Answer from the drawing. Dimensions are ordinates in mm from the lowest x, y and z of the part. Give positions to 0.01 mm unless a question says otherwise; leave off trailing zeros. Write each loop counter-clockwise with the first axis right and the second up, starting at its lowest first coordinate (ties: lowest second). Pieces come first, ordered by that corner, then holes. Notation, with made-up numbers: M -39.75,16.25 L -26.75,16.25 A10 ccw -26.75,32.25 Z; hole C 1,39.25 d6. An arc over 180 degrees is marked long. Answer as a JSON object with one key per item and string values.
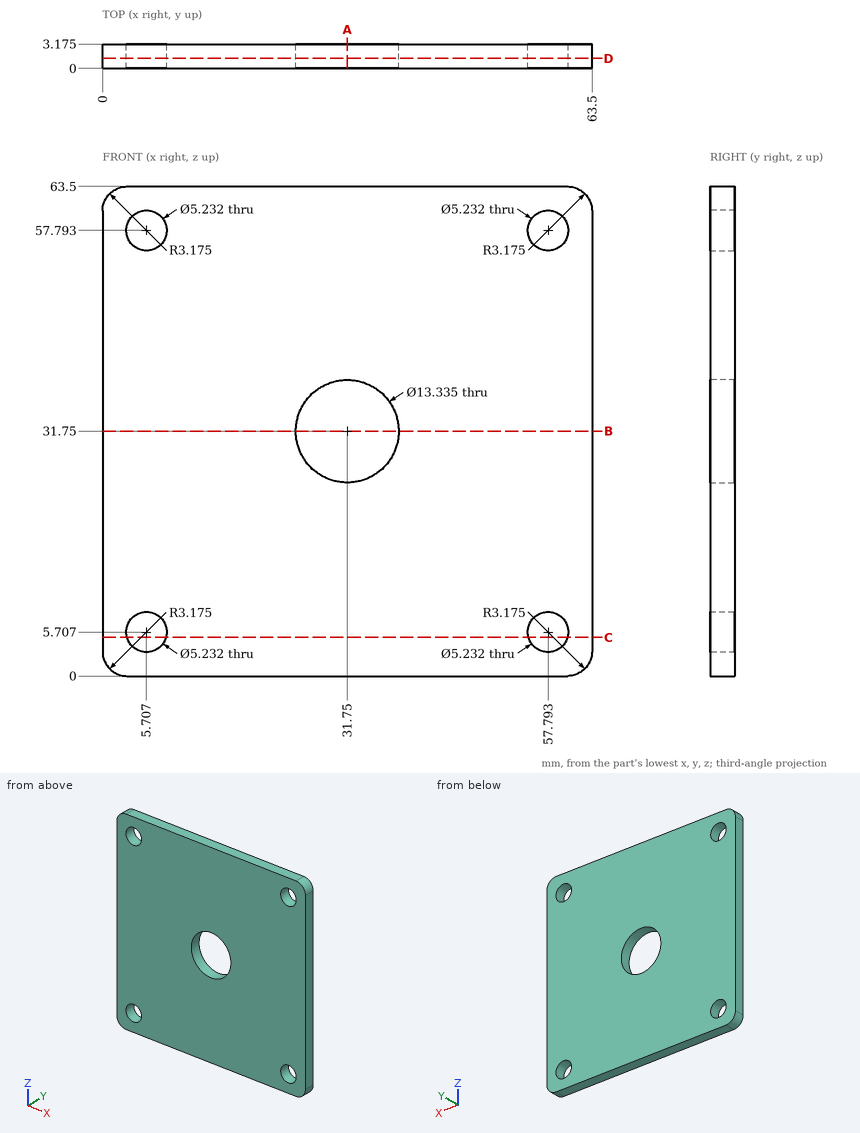
1. A cutting plane is placed at C-C, the plane z = 5. Give the vertices of the cut face in (x, y) (1 decimal).
Verdict:
{"outline": "M 0,0 L 3.2,0 L 3.2,3.2 L 0,3.2 Z; M 8.2,0 L 55.3,0 L 55.3,3.2 L 8.2,3.2 Z; M 60.3,0 L 63.5,0 L 63.5,3.2 L 60.3,3.2 Z"}
2. Consider line 1 along X through (y, z) = (0.2, 31.5); line 2 along Z through (x, y) = (7.5, 0.15) (1 decimal); line 3 along X through (y, z) = (1.1, 7). Determine where each line is inside the solid, lowest interval first.
Verdict:
{"line 1": "x = 0 to 25.09, 38.41 to 63.5", "line 2": "z = 0 to 3.8, 7.6 to 55.9, 59.7 to 63.5", "line 3": "x = 0 to 3.43, 7.98 to 55.52, 60.07 to 63.5"}
3. A cutting plane is placed at D-D, the plane y = 1.3. Count the separate pieces of the cut face and the enclosed holes in it, plus the area to 3 significant figures.
Verdict:
{"separate pieces": "1", "enclosed holes": "5", "area": "3,800 mm2"}
4. A flat-ended cylindrical pin translates along its axis: pin 1 (4 mm diameter, centred on x = 57.79, z = 5.71, fed in from -Y). Find the tip coordinate at first contact, or state that the pin passes through.
Verdict:
{"pin 1": "passes through"}
5. A cutting plane is placed at A-A, the plane x = 31.75. Give the vertices of the cut face in (y, z) (1 decimal), plus the area to 3 significant figures.
Verdict:
{"outline": "M 0,0 L 3.2,0 L 3.2,25.1 L 0,25.1 Z; M 0,38.4 L 3.2,38.4 L 3.2,63.5 L 0,63.5 Z", "area": "159 mm2"}
6. A cutting plane is placed at B-B, the plane z = 31.75. Give the vertices of the cut face in (x, y) (1 decimal), plus the area to 3 significant figures.
Verdict:
{"outline": "M 0,0 L 25.1,0 L 25.1,3.2 L 0,3.2 Z; M 38.4,0 L 63.5,0 L 63.5,3.2 L 38.4,3.2 Z", "area": "159 mm2"}
